```python
from build123d import *

# Parameters (mm, degrees)
F0_R     = 12.7
F1_DEPTH = 88.9
F2_R     = 6.35
F3_DEPTH = 38.1
F4_R     = 6.35
F5_DEPTH = 25.4


with BuildPart() as f1:
    # F0 (on Front) → F1 (new body)
    with BuildSketch(Plane.XZ):
        Circle(F0_R)
    extrude(amount=-F1_DEPTH)

    # F2 (on face) → F3 (join)
    with BuildSketch(Plane(origin=(0, 88.9, 0), x_dir=(-1, 0, 0), z_dir=(0, 1, 0))):
        Circle(F2_R)
    extrude(amount=F3_DEPTH)

    # F4 (on Right) → F5 (join)
    with BuildSketch(Plane.YZ):
        with Locations((127, 0)):
            Circle(F4_R)
    extrude(amount=F5_DEPTH)


solid = f1.part
```
Work out the finished part from the listing and answer in its coordinate system (mm). A direction names the side the tool comes from. Round coordinates to 2 decimals unless told otherwise and drop trailing zeros. Write each loop counter-clockwise with the first axis right and the second up, starting at its lowest first coordinate (ties: lowest second). Pieces come first, ordered by that corner, then holes. Notation, with made-up numbers: (62, -8) -> (96, -8) arc R19 cw to (96, 8) -> close; hole circle Ø3 at (83, 80.5). An arc over 180 degrees is marked (long way). Write each question's results on one line, items separated by ' | '.
Q1. Section A-A, the plane z = 0 is taken. Write down the section's boundary in (x, y), then the cut area to 3 significant figures.
Data:
outline: (-12.7, 0) -> (12.7, 0) -> (12.7, 88.9) -> (6.35, 88.9) -> (6.35, 120.65) -> (25.4, 120.65) -> (25.4, 133.35) -> (0, 133.35) -> (0, 127) -> (-6.35, 127) -> (-6.35, 88.9) -> (-12.7, 88.9) -> close | area: 3,020 mm^2
Q2. Determine the mould class of faces 4 (the flat face through (0, 129, 0)), 5 (the cylindrical face through (-6.057, 107.683, 1.907)), 6 (the flat face through (0, 0, 0)) for opening direction Y: released by +Y, released by -Y, zero draft, split by the parting line, or undercut.
Data:
face 4: zero draft | face 5: undercut | face 6: released by -Y
Q3. Straight lines are drawn through the part: line 1 along Y through (x, z) = (-5, 1.25); line 2 along Y through (x, z) = (-6, -8.5); line 3 along Y through (x, z) = (7.5, 5.75). For each, find the intervals that lie inside material, in ascending order. Write a range as [from, to].
Data:
line 1: [0, 127] | line 2: [0, 88.9] | line 3: [0, 88.9], [124.31, 129.69]
Q4. Section D-D, the plane y = 101 is taken. Write down the section's boundary in (x, z).
Data:
outline: circle Ø12.7 at (0, 0)
Q5. Section C-C, the plane x = -5 is taken. Write down the section's boundary in (y, z).
Data:
outline: (0, -11.67) -> (88.9, -11.67) -> (88.9, -3.91) -> (127, -3.91) -> (127, 3.91) -> (88.9, 3.91) -> (88.9, 11.67) -> (0, 11.67) -> close
Q6. Which of the six approach directions +Z, -Z, +X, -X, +Y, -Y give full straight-line access (tool end or side, diameter ignored) to faces 1 (the cylindrical face through (-2.75, 43.83, -12.4)), 2 (the cylindrical face through (12.522, 133.057, 1.907)), 3 (the flat face through (3, 88.9, 6))?
Data:
face 1: -Y | face 2: +X | face 3: none
Q7. Flat-ended cylindrical pins translate along their axes: P1, Ø1, axis at x = -7.5, z = -3.5, coming from the -Y side; P2, Ø6, axis at x = -8.5, y = 52.5, coming from the -Z side; P3, Ø5, axis at y = 130, z = 3, coming from the -X side; P4, Ø7, axis at x = -4, z = -0.5, coming from the +Y side. Find the tip coordinate at first contact, or state that the pin passes through.
Data:
P1: y = 0 | P2: z = -11.45 | P3: x = 0 | P4: y = 127
Q8. Section B-B, the plane x = 8 is taken. Write down the section's boundary in (y, z).
Data:
outline: (0, -9.86) -> (88.9, -9.86) -> (88.9, 9.86) -> (0, 9.86) -> close; circle Ø12.7 at (127, 0)
